from build123d import *

# Parameters (mm, degrees)
SKETCH_1_R          = 2.5
EXTRUDE_1_DEPTH     = 10
SKETCH_2_R          = 2.5
CUT_EXTRUDE_1_DEPTH = 20
CHAMFER_1_SIZE      = 4
FILLET_1_R          = 0.2


with BuildPart() as part:
    # Эскиз1 → Вытянуть1 (new body)
    with BuildSketch(Plane.XY):
        Polygon((17.000000013, -23.429402734), (17.000000013, -12.754084516), (4.776542266, -12.754084516), (4.776542266, -4.5), (-4.5, -4.5), (-4.5, 4.5), (25.000000013, 4.5), (25.000000013, -23.429402734), align=None)
        Circle(SKETCH_1_R, mode=Mode.SUBTRACT)
    extrude(amount=EXTRUDE_1_DEPTH)

    # Эскиз2 → Вырез-Вытянуть1 (cut)
    with BuildSketch(Plane.XZ.offset(23.429402734)):
        with Locations(Location((21.000000013, 5, 0), (0, 0, 270))):
            Circle(SKETCH_2_R)
    extrude(amount=-CUT_EXTRUDE_1_DEPTH, mode=Mode.SUBTRACT)

    # Фаска1
    chamfer_1_edges = [part.edges().sort_by_distance(p)[0] for p in [
        (25.000000013, 4.5, 5),
    ]]
    chamfer(chamfer_1_edges, length=CHAMFER_1_SIZE)

    # Скругление1
    fillet_1_edges = [part.edges().sort_by_distance(p)[0] for p in [
        (10.88827114, -12.754084516, 10),
        (17.000000013, -18.091743625, 10),
        (17.000000013, -18.091743625, 0),
        (10.88827114, -12.754084516, 0),
    ]]
    fillet(fillet_1_edges, radius=FILLET_1_R)


solid = part.part
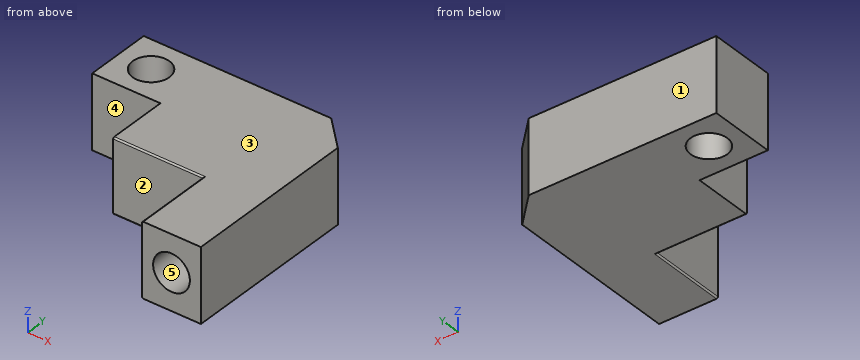
The model under review builds one solid part; all positions refer to its coordinate system, in mm. Face numbers are marked on the shaded views. A direction names the side the tool comes from. Round coordinates to 2 decimals unless told otherwise and drop trailing zeros. Write each loop counter-clockwise with the first axis right and the second up, starting at its lowest first coordinate (ties: lowest second). Pieces come first, ordered by that corner, then holes. Notation, with made-up numbers: M -36,-36.5 L -15,-36.5 A28 ccw -15,-15.5 Z; hole C -4.5,50 d2. An arc over 180 degrees is marked long. Answer as CSV lines item,"result". Start each with the question number.
Q1. Wall thickness on line 1 along Y through (x, z) = (0, 2.5); line 2 along X through (y, z) = (-16.5, 5); line 3 along X through (y, z) = (-8, 6): over which ranges is each line inside the solid? List them lowest first.
Q2. The part is to be moulded in two halves that separate along Z. For the marked faces 3, 4 and 5, say which applies: +Z half, -Z half, draft (parallel to the pull), parting line (faces both ways), or undercut.
Q3. Consider section D-D, the plane y = -18. Give the boundary of the cut face in (x, z), then the cut area to 3 significant figures.
Q4. Consider section C-C, the plane x = -0.75. Give the boundary of the cut face in (y, z).
Q5. Consider section B-B, the plane y = 0. Give the boundary of the cut face in (x, z).
Q6. Tool access review of the marked faces 1 and 2: name each direction out of +Z, -Z, +X, -X, +Y, -Y from which nothing blocks a thin tool from reaching the whole face with its end or side.
Q7. Consider section A-A, the plane z = 8. Give the boundary of the cut face in (x, y), then the cut area to 3 significant figures.
Q8. Clearance check with flat-ended pins moving along their axes: P1, Ø3, axis at x = 21, z = 5, coming from the -Y side; P2, Ø2.5, axis at y = -9, z = 4.5, coming from the -X side. State where each tip first meets the part, or that it passes through.
Result set:
1,line 1,"y = -4.5 to -2.5, 2.5 to 4.5"
1,line 2,"x = 17 to 18.5, 23.5 to 25"
1,line 3,"x = 4.78 to 18.71, 23.29 to 25"
2,face 3,"+Z half"
2,face 4,"draft"
2,face 5,"undercut"
3,outline,"M 17,0.2 A0.2 ccw 17.2,0 L 25,0 L 25,10 L 17.2,10 A0.2 ccw 17,9.8 Z; hole C 21,5 d5"
3,area,"60.3 mm²"
4,outline,"M -4.5,0 L -2.38,0 L -2.38,10 L -4.5,10 Z; M 2.38,0 L 4.5,0 L 4.5,10 L 2.38,10 Z"
5,outline,"M -4.5,0 L -2.5,0 L -2.5,10 L -4.5,10 Z; M 2.5,0 L 25,0 L 25,10 L 2.5,10 Z"
6,face 1,"+Z, -Z, +X, -X, +Y"
6,face 2,"+Z, -Z, -X, -Y"
7,outline,"M -4.5,-4.5 L 4.78,-4.5 L 4.78,-12.75 L 17,-12.75 L 17,-23.43 L 25,-23.43 L 25,0.5 L 21,4.5 L -4.5,4.5 Z; hole C 0,0 d5"
7,area,"490 mm²"
8,P1,"stops at y = -3.43"
8,P2,"stops at x = 4.78"
